Build history of the part. All positions in model axes, mm. A direction names the side the tool comes from. Round coordinates to 2 decimals unless told otherwise and drop trailing zeros. Order: outer loops, then holes, each group sorted by start corner. A loop starts at its lowest first (then second) coordinate and runs counter-clockwise, first axis right, second up. Notation, with made-up numbers: (-2.5, 16.25) -> (26.5, 16.25) arc R15 ccw to (26.5, 37.25) -> close; hole circle Ø1 at (66.25, 58). An arc over 180 degrees is marked (long way). Write item = value, one per line.
from build123d import *

# Parameters (mm, degrees)
BOX_W                              = 235
BOX_H                              = 30
BOX_DEPTH                          = 117
SKETCH_W                           = 75
SKETCH_H                           = 25
POCKET_DEPTH                       = 115.5
POCKET001_DEPTH                    = 300
SKETCH002_W                        = 75
SKETCH002_H                        = 7
POCKET002_DEPTH                    = 5
SKETCH002_LINEARPATTERN001_2_W     = 75
SKETCH002_LINEARPATTERN001_2_H     = 7
POCKET002_LINEARPATTERN001_2_DEPTH = 5
SKETCH002_LINEARPATTERN001_3_W     = 75
SKETCH002_LINEARPATTERN001_3_H     = 7
POCKET002_LINEARPATTERN001_3_DEPTH = 5
LINEARPATTERN002_COUNT             = 3
LINEARPATTERN002_PITCH             = 8.5
FILLET_R                           = 0.5
SKETCH003_W                        = 235
SKETCH003_H                        = 9
PAD_DEPTH                          = 10
POCKET003_DEPTH                    = 235.001


with BuildPart() as part:
    # Box → Box (new body)
    with BuildSketch(Plane.XY):
        with Locations((117.5, 15)):
            Rectangle(BOX_W, BOX_H)
    extrude(amount=BOX_DEPTH)

    # Sketch (on Face6 of BaseFeature) → Pocket (cut)
    with BuildSketch(Plane.XY.offset(117)):
        with Locations((40, 15)):
            Rectangle(SKETCH_W, SKETCH_H)
        with Locations((117.5, 15)):
            Rectangle(SKETCH_W, SKETCH_H)
        with Locations((195, 15)):
            Rectangle(SKETCH_W, SKETCH_H)
    extrude(amount=-POCKET_DEPTH, mode=Mode.SUBTRACT)

    # Sketch001 (on Face6 of Pocket) → Pocket001 (cut)
    with BuildSketch(Plane.YZ.offset(235)):
        Polygon((10, 117), (30, 40), (40, 120), align=None)
    extrude(amount=-POCKET001_DEPTH, mode=Mode.SUBTRACT)

    # Sketch002 (on Face5 of Pocket001) → Pocket002 (cut)
    with BuildSketch(Plane(origin=(0, 0, 0), x_dir=(1, 0, 0), z_dir=(0, 0, -1))):
        with Locations((40, -6)):
            Rectangle(SKETCH002_W, SKETCH002_H)
    pocket002 = extrude(amount=-POCKET002_DEPTH, mode=Mode.SUBTRACT)

    # Sketch002 LinearPattern001 2 → Pocket002 LinearPattern001 2 (cut)
    with BuildSketch(Plane(origin=(77.5, 0, 0), x_dir=(1, 0, 0), z_dir=(0, 0, -1))):
        with Locations((40, -6)):
            Rectangle(SKETCH002_LINEARPATTERN001_2_W, SKETCH002_LINEARPATTERN001_2_H)
    pocket002_linearpattern001_2 = extrude(amount=-POCKET002_LINEARPATTERN001_2_DEPTH, mode=Mode.SUBTRACT)

    # Sketch002 LinearPattern001 3 → Pocket002 LinearPattern001 3 (cut)
    with BuildSketch(Plane(origin=(155, 0, 0), x_dir=(1, 0, 0), z_dir=(0, 0, -1))):
        with Locations((40, -6)):
            Rectangle(SKETCH002_LINEARPATTERN001_3_W, SKETCH002_LINEARPATTERN001_3_H)
    pocket002_linearpattern001_3 = extrude(amount=-POCKET002_LINEARPATTERN001_3_DEPTH, mode=Mode.SUBTRACT)

    # LinearPattern002: Pocket002, Pocket002 LinearPattern001 2, Pocket002 LinearPattern001 3 ×3
    with Locations(*[(0, i * LINEARPATTERN002_PITCH, 0) for i in range(1, LINEARPATTERN002_COUNT)]):
        add(pocket002, mode=Mode.SUBTRACT)
        add(pocket002_linearpattern001_2, mode=Mode.SUBTRACT)
        add(pocket002_linearpattern001_3, mode=Mode.SUBTRACT)

    # Fillet
    fillet_edges = [part.edges().sort_by_distance(p)[0] for p in [
        (117.5, 30, 40),
        (117.5, 30, 0),
        (0, 30, 20),
        (0, 20, 78.5),
        (2.5, 18.75, 83.3125),
        (40, 27.5, 49.625),
        (77.5, 18.75, 83.3125),
        (80, 18.75, 83.3125),
        (117.5, 27.5, 49.625),
        (155, 18.75, 83.3125),
        (157.5, 18.75, 83.3125),
        (195, 27.5, 49.625),
        (232.5, 18.75, 83.3125),
        (235, 20, 78.5),
        (235, 30, 20),
        (1.25, 10, 117),
        (78.75, 10, 117),
        (156.25, 10, 117),
        (233.75, 10, 117),
        (195, 2.5, 117),
        (40, 2.5, 117),
        (117.5, 2.5, 117),
    ]]
    fillet(fillet_edges, radius=FILLET_R)

    # Sketch003 (on Face4 of Fillet) → Pad (join)
    with BuildSketch(Plane.XZ):
        with Locations((117.5, 112.5)):
            Rectangle(SKETCH003_W, SKETCH003_H)
        with Locations((117.5, 4.5)):
            Rectangle(SKETCH003_W, SKETCH003_H)
    extrude(amount=PAD_DEPTH)

    # Sketch004 (on Face76 of Pad) → Pocket003 (cut, through all)
    with BuildSketch(Plane.YZ.offset(235)):
        with BuildLine():
            ThreePointArc((-5.478476, 114.999907), (-7.903779, 111.813088), (-4.160827, 110.38893))
            Line((-4.160827, 105.760277), (-4.160827, 110.38893))
            Line((0, 105.760277), (-4.160827, 105.760277))
            Line((0, 114.999907), (0, 105.760277))
            Line((-5.478476, 114.999907), (0, 114.999907))
        make_face()
        with BuildLine():
            ThreePointArc((-4.401101, 6.745533), (-7.935553, 5.063989), (-5.5, 2))
            Line((-5.5, 2), (0, 2))
            Line((0, 2), (-0.240678, 13.918851))
            Line((-0.240678, 13.918851), (-4.401101, 13.860906))
            Line((-4.401101, 13.860906), (-4.401101, 6.745533))
        make_face()
    extrude(amount=-POCKET003_DEPTH, mode=Mode.SUBTRACT)


solid = part.part
Q1. Mould opens along X. For faces 1 (the face through (79.85, 19.217, 80.946)), 2 (the face through (118.046, 28.833, 44.494)), 3 (the face through (0.143, 19.69, 79.095)), 4 (the face through (235, 10, 45)) say: released by +X, released by -X, zero draft, split by the parting line, or undercut.
Check values:
face_1 = undercut
face_2 = zero draft
face_3 = released by -X
face_4 = released by +X
Q2. Cut at A-A, the plane x = 109. Give the number of separate pieces and of enclosed holes in the cut face, and give its area (3 significant figures).
Check values:
separate_pieces = 4
enclosed_holes = 0
area = 498 mm²
Q3. Flat gauge pins, fed straight in: pin 1 (0.8 mm diameter, centred on x = 133, y = 10, fed in from +Z); pin 2 (1.5 mm diameter, centred on x = 202, z = 73.5, fed in from -Y); pin 3 (1 mm diameter, centred on x = 182.5, z = 91.5, fed in from +Y); pin 4 (5 mm diameter, centred on y = 16, z = 105, fed in from +X). Where does each tip first touch, or does it go through?
Check values:
pin_1 = 1.5
pin_2 = 0
pin_3 = 2.5
pin_4 = through
Q4. Probe probe 1 along Y at (x, z) = (180, 4); probe 2 along X at (y, z) = (15.5, 90); probe 3 along Z at (x, y) = (130, -5.5). List the from-to ranges inside material, lowest first.
Check values:
probe_1 = -10 to -7.95, -0.04 to 2.5, 27.5 to 30
probe_2 = 0 to 2.5, 77.5 to 80, 155 to 157.5, 232.5 to 235
probe_3 = 0 to 2, 7 to 9, 108 to 110, 115 to 117
Q5. Cut at B-B, the plane z = 14. List the corners of the cut face in (x, y).
Check values:
outline = (0, 0) -> (235, 0) -> (235, 29.5) arc R0.5 ccw to (234.5, 30) -> (0.5, 30) arc R0.5 ccw to (0, 29.5) -> close; hole (2.5, 2.5) -> (77.5, 2.5) -> (77.5, 27.5) -> (2.5, 27.5) -> close; hole (80, 2.5) -> (155, 2.5) -> (155, 27.5) -> (80, 27.5) -> close; hole (157.5, 2.5) -> (232.5, 2.5) -> (232.5, 27.5) -> (157.5, 27.5) -> close
Q6. Which spindle directions (+Z, -Z, +X, -X, +Y, -Y) get a long thin tool onto all of the face, cutting with end or side? Do faces 5 (the face through (194, 27.5, 24)), 6 (the face through (157.35, 19.217, 80.946)), 7 (the face through (117, 2.5, 57)). Say none if no direction does.
Check values:
face_5 = +Z
face_6 = +Z, +Y
face_7 = +Z, -Z
